Here's how the part is built. I have some questions about the finished solid (model axes, mm). A direction names the side the tool comes from. Give positions to 0.01 mm unless a question says otherwise; leave off trailing zeros. Write each loop counter-clockwise with the first axis right and the second up, starting at its lowest first coordinate (ties: lowest second). Pieces come first, ordered by that corner, then holes. Notation, with made-up numbers: M -18.75,51 L 28.25,51 A18 ccw 28.25,75 Z; hole C 55,9.25 d6. An arc over 180 degrees is marked long. Use one line per item in the form item = value. Start each with the question number.
from build123d import *

# Parameters (mm, degrees)
F0_W     = 5
F0_H     = 8
F1_DEPTH = 4
F2_R     = 1.99999


# Not quite as in the source:
# - a fillet or chamfer is up to 0.001 mm smaller than in the source, because OpenCascade refuses the exact size


with BuildPart() as f1:
    # F0 (on Top) → F1 (new body)
    with BuildSketch(Plane.XY):
        Polygon((-2.5, 2), (-40, 2), (-40, -2), (40, -2), (40, 2), (2.5, 2), align=None)
        with Locations((0, 6)):
            Rectangle(F0_W, F0_H)
    extrude(amount=F1_DEPTH)

    # F2 (radius 2 in the source; OpenCascade refuses exactly that, so slightly less here)
    f2_edges = [f1.edges().sort_by_distance(p)[0] for p in [
        (-40, -2, 2),
        (40, -2, 2),
        (40, 2, 2),
        (-40, 2, 2),
        (-2.5, 10, 2),
        (2.5, 10, 2),
        (-2.5, 2, 2),
        (2.5, 2, 2),
    ]]
    fillet(f2_edges, radius=F2_R)


solid = f1.part
1) Suppose I cut it at C-C, the plane y = 6. List the corners of the cut face in (x, z) for me.
2) Please list where these lines run through material, in increasing order: line 1 (Y direction, x = -27.5, z = 0.4); line 2 (X direction, y = 5, z = 3.1); line 3 (X direction, y = 1, z = 0.95).
3) Suppose I cut it at B-B, the plane x = 8.5. List the corners of the cut face in (y, z) for me.
4) On a 3-axis mill with a long thin cutter (end or side, diameter ignored), from which of +Z, -Z, +X, -X, +Y, -Y can I reach the whole of each face in a straight line? I mean faces 1 (the face through (2.5, 6, 2)), 2 (the face through (-21, 2, 2)), 3 (the face through (-39.43, -1.4, 2.03)). Say none if no direction works.
5) Will these pins go through, and if not, where does the flat tip stop? P1, Ø2, axis at x = 31.5, z = 2, coming from the +Y side; P2, Ø2, axis at y = 6, z = 2, coming from the -X side; P3, Ø1, axis at y = 8.5, z = 0.5, coming from the +X side; P4, Ø4, axis at x = 31.5, y = 3.5, coming from the +Z side.
Checks:
q1.outline = M -2.5,0 L 2.5,0 L 2.5,4 L -2.5,4 Z
q2.line_1 = -2 to 2
q2.line_2 = -2.5 to 2.5
q2.line_3 = -39.73 to 39.73
q3.outline = M -2,0 L 2,0 L 2,4 L -2,4 Z
q4.face_1 = +Z, -Z, +X, +Y
q4.face_2 = +Z, -Z, -X, +Y
q4.face_3 = +Z, -Z, -X, -Y
q5.P1 = 2
q5.P2 = -2.5
q5.P3 = 2.5
q5.P4 = 4
